from build123d import *

# Parameters (mm, degrees)
F0_W     = 30
F0_H     = 90
F1_DEPTH = 370
F2_T     = -3
F3_R     = 2.5527
F3_R_2   = 14.28115
F3_R_3   = 8.3312
F4_DEPTH = 30.001
F5_R     = 4
F6_DEPTH = 30.001


# Not quite as in the source:
# - a pattern or mirror of a feature is missing from the dataset's text; its kind, count and spacing are read off the source's solid


with BuildPart() as f1:
    # F0 (on Front) → F1 (new body, symmetric)
    with BuildSketch(Plane.XZ):
        Rectangle(F0_W, F0_H)
    extrude(amount=F1_DEPTH, both=True)

    # F2
    f2_openings = [f1.faces().sort_by_distance(p)[0] for p in [
        (0, -370, 0),
        (0, 370, 0),
    ]]
    offset(amount=F2_T, openings=f2_openings)

    # F3 (on face) → F4 (cut, through all)
    with BuildSketch(Plane.YZ.offset(15)):
        with Locations((228.1688, 36.5125)):
            Circle(F3_R)
        with Locations((228.1688, -36.5125)):
            Circle(F3_R)
        with Locations((285.3188, -36.5125)):
            Circle(F3_R)
        with Locations((285.3188, 36.5125)):
            Circle(F3_R)
        with Locations((256.7438, 0)):
            Circle(F3_R_2)
        with Locations((213.4876, 0)):
            Circle(F3_R_3)
        with Locations((300, 0)):
            Circle(F3_R_3)
    f4 = extrude(amount=-F4_DEPTH, mode=Mode.SUBTRACT)

    # F4_copies: F4 across plane
    add(f4.mirror(Plane(origin=(0, 0, 0), x_dir=(0, 0, -1), z_dir=(0, -1, 0))), mode=Mode.SUBTRACT)

    # F5 (on face) → F6 (cut, through all)
    with BuildSketch(Plane.YZ.offset(15)):
        with Locations((-338, 37)):
            Circle(F5_R)
        with Locations((-350, 0)):
            Circle(F5_R)
        with Locations((-338, -37)):
            Circle(F5_R)
    f6 = extrude(amount=-F6_DEPTH, mode=Mode.SUBTRACT)

    # F6_copies: F6 across plane
    add(f6.mirror(Plane.ZX), mode=Mode.SUBTRACT)


solid = f1.part
Model file for the job. Use its own axes, mm. A direction names the side the tool comes from. Round coordinates to 2 decimals unless told otherwise and drop trailing zeros. Loops run counter-clockwise (first coordinate to the right, second up) from the corner with the lowest first, then second, coordinate; pieces in that order, holes last. Notation, with made-up numbers: M 25,37.25 L 49,37.25 A23 ccw 49,76.25 Z; hole C 89,35.25 d11. An arc over 180 degrees is marked long. One line per question, with ' | ' between items.
1) 3-axis set-ups, long thin cutter, end or side, ignore diameter. For faces 4 (the flat face through (-15, -5, -1)), 5 (the flat face through (-12, -5, -1)): which of +Z, -Z, +X, -X, +Y, -Y reach the whole face in a straight line?
Solved:
face 4: +Z, -Z, -X, +Y, -Y | face 5: +Y, -Y
2) Band-saw the part on B-B (y = 300). Give the cut face in (x, z), then the cut area to 3 significant figures.
Solved:
outline: M -15,-45 L 15,-45 L 15,-8.33 L 12,-8.33 L 12,-42 L -12,-42 L -12,-8.33 L -15,-8.33 Z; M -15,8.33 L -12,8.33 L -12,42 L 12,42 L 12,8.33 L 15,8.33 L 15,45 L -15,45 Z | area: 584 mm²
3) Mould opens along Y. For faces 1 (the flat face through (0, -5, -45)), 2 (the cylindrical face through (-13.479, -270.365, 4.29)), 3 (the flat face through (-12.3, -370, 3.5)) say: +Y half, -Y half, draft (parallel to the pull), parting line (faces both ways), or undercut.
Solved:
face 1: draft | face 2: undercut | face 3: -Y half
4) Band-saw the part on A-A (x = 0). Give the cut face in (y, z).
Solved:
outline: M -370,-45 L 370,-45 L 370,-42 L -370,-42 Z; M -370,42 L 370,42 L 370,45 L -370,45 Z
5) Band-saw the part on D-D (y = 0). Give the cut face in (x, z), then the cut area to 3 significant figures.
Solved:
outline: M -15,-45 L 15,-45 L 15,45 L -15,45 Z; hole M -12,-42 L 12,-42 L 12,42 L -12,42 Z | area: 684 mm²
6) Band-saw the part on C-C (z = 20.5). Give the cut face in (x, y).
Solved:
outline: M -15,-370 L -12,-370 L -12,370 L -15,370 Z; M 12,-370 L 15,-370 L 15,370 L 12,370 Z
7) Drill centre lines: line 1 along X through (y, z) = (-271, -20.5); line 2 along Z through (x, y) = (1, 119); line 3 along Z through (x, y) = (13.55, 300). Where is each one in solid material? Low to high.
Solved:
line 1: x = -15 to -12, 12 to 15 | line 2: z = -45 to -42, 42 to 45 | line 3: z = -45 to -8.33, 8.33 to 45
